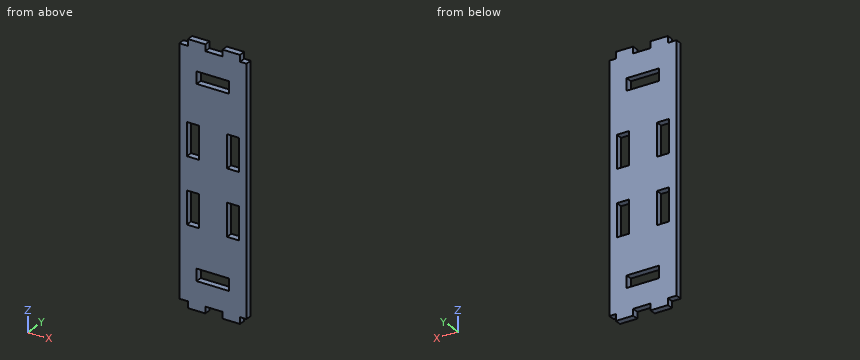
from build123d import *

# Parameters (mm, degrees)
SKETCH1_W           = 15
SKETCH1_H           = 5.5
SKETCH1_W_2         = 5.5
SKETCH1_H_2         = 15
BOSS_EXTRUDE1_DEPTH = 3


with BuildPart() as part:
    # Sketch1 → Boss-Extrude1 (new body)
    with BuildSketch(Plane(origin=(0, 0, 0), x_dir=(1, 0, 0), z_dir=(0, 1, 0))):
        Polygon((0, 56), (0, -56), (-3, -56), (-3, -59), (-11, -59), (-11, -56), (-19, -56), (-19, -59), (-27, -59), (-27, -56), (-31, -56), (-31, 56), (-27, 56), (-27, 59), (-19, 59), (-19, 56), (-11, 56), (-11, 59), (-3, 59), (-3, 56), align=None)
        with Locations((-15.5, -43.25)):
            Rectangle(SKETCH1_W, SKETCH1_H, mode=Mode.SUBTRACT)
        with Locations((-24.75, -15)):
            Rectangle(SKETCH1_W_2, SKETCH1_H_2, mode=Mode.SUBTRACT)
        with Locations((-6.25, -15)):
            Rectangle(SKETCH1_W_2, SKETCH1_H_2, mode=Mode.SUBTRACT)
        with Locations((-24.75, 15)):
            Rectangle(SKETCH1_W_2, SKETCH1_H_2, mode=Mode.SUBTRACT)
        with Locations((-6.25, 15)):
            Rectangle(SKETCH1_W_2, SKETCH1_H_2, mode=Mode.SUBTRACT)
        with Locations((-15.5, 43.25)):
            Rectangle(SKETCH1_W, SKETCH1_H, mode=Mode.SUBTRACT)
    extrude(amount=BOSS_EXTRUDE1_DEPTH)


solid = part.part
Input: part model. Units: mm. Frame: model coordinates. Give positions to 0.01 mm unless a question says otherwise; leave off trailing zeros. Order: outer loops, then holes, each group sorted by start corner. A loop starts at its lowest first (then second) coordinate and runs counter-clockwise, first axis right, second up. Notation, with made-up numbers: M 8,67 L 66,67 A27 cw 66,100 Z; hole C 62,43.5 d6. An arc over 180 degrees is marked long. Answer as a JSON object with one key per item and string values.
1. Ray query, line 1 (Z direction, x = -24.5, y = 2.75); line 2 (Z direction, x = -18, y = 1.7); line 3 (X direction, y = 2.6, z = -12.5). Return the intervals inside material, ascending. Write a range as [from, to].
Result sheet:
{"line 1": "[-59, -22.5], [-7.5, 7.5], [22.5, 59]", "line 2": "[-56, -46], [-40.5, 40.5], [46, 56]", "line 3": "[-31, -27.5], [-22, -9], [-3.5, 0]"}
2. Cut plane C-C, the plane y = 2.45. State how many separate pieces and enclosed holes the cut face has, and give its area (3 significant figures).
Result sheet:
{"separate pieces": "1", "enclosed holes": "6", "area": "3,070 mm²"}
3. Cut plane B-B, the plane x = -5. Output: boundary loops of the cut face in (y, z), and give its area (3 significant figures).
Result sheet:
{"outline": "M 0,-59 L 3,-59 L 3,-22.5 L 0,-22.5 Z; M 0,-7.5 L 3,-7.5 L 3,7.5 L 0,7.5 Z; M 0,22.5 L 3,22.5 L 3,59 L 0,59 Z", "area": "264 mm²"}
4. First-contact query: P1, Ø1.5, axis at y = 1, z = -57.5, coming from the +X side; P2, Ø1.5, axis at y = 1, z = 57, coming from the -X side. Flat tips, straight axial feed; report the tip coordinate or a pass-through.
Result sheet:
{"P1": "x = -3", "P2": "x = -27"}
5. Cut plane A-A, the plane z = -19. Output: boundary loops of the cut face in (x, y).
Result sheet:
{"outline": "M -31,0 L -27.5,0 L -27.5,3 L -31,3 Z; M -22,0 L -9,0 L -9,3 L -22,3 Z; M -3.5,0 L 0,0 L 0,3 L -3.5,3 Z"}
